```python
from build123d import *

# Parameters (mm, degrees)
SKETCH1_R           = 50
BOSS_EXTRUDE1_DEPTH = 20
CUT_EXTRUDE3_DEPTH  = 74.484692283
SKETCH14_W          = 22.5
SKETCH14_H          = 12.2
CUT_EXTRUDE4_DEPTH  = 74.484692283
SKETCH16_W          = 4.8
SKETCH16_H          = 12.2
CUT_EXTRUDE5_DEPTH  = 11.25
CUT_EXTRUDE7_START  = -11.25
SKETCH17_R          = 0.5
CUT_EXTRUDE7_DEPTH  = 0.4
CUT_EXTRUDE8_DEPTH  = 74.484692283
FILLET1_R           = 2
FILLET2_R           = 0.5
SKETCH4_R           = 14
CUT_EXTRUDE2_DEPTH  = 74.484692283
SKETCH20_W          = 4.8
SKETCH20_H          = 12.2
BOSS_EXTRUDE2_DEPTH = 4
FILLET3_R           = 10


with BuildPart() as part:
    # Sketch1 → Boss-Extrude1 (new body)
    with BuildSketch(Plane(origin=(0, 0, 0), x_dir=(1, 0, 0), z_dir=(0, 1, 0))):
        with Locations(Location((0, 0, 0), (0, 0, 270))):
            Circle(SKETCH1_R)
    extrude(amount=BOSS_EXTRUDE1_DEPTH)

    # Sketch15 → Cut-Extrude3 (cut, through all)
    with BuildSketch(Plane.XZ):
        with BuildLine():
            Line((-21.2, 6.1), (-21.2, 45.283109434))
            ThreePointArc((-21.2, 45.283109434), (-5.873377692, 49.65383605), (10.05, 48.979562064))
            Line((10.05, 48.979562064), (10.9, 6.1))
            Line((10.9, 6.1), (-21.2, 6.1))
        make_face()
    extrude(amount=-CUT_EXTRUDE3_DEPTH, mode=Mode.SUBTRACT)

    # Sketch14 → Cut-Extrude4 (cut, through all)
    with BuildSketch(Plane.XZ):
        with Locations((-5.15, 0)):
            Rectangle(SKETCH14_W, SKETCH14_H)
    extrude(amount=-CUT_EXTRUDE4_DEPTH, mode=Mode.SUBTRACT)

    # Sketch16 → Cut-Extrude5 (cut)
    with BuildSketch(Plane.XZ):
        with Locations((-18.8, 0)):
            Rectangle(SKETCH16_W, SKETCH16_H)
        with Locations((8.5, 0)):
            Rectangle(SKETCH16_W, SKETCH16_H)
    extrude(amount=-CUT_EXTRUDE5_DEPTH, mode=Mode.SUBTRACT)

    # Sketch17 → Cut-Extrude7 (cut)
    with BuildSketch(Plane.XZ.offset(CUT_EXTRUDE7_START)):
        with Locations(Location((8.75, 0, 0), (0, 0, 270))):
            Circle(SKETCH17_R)
        with Locations(Location((-19.05, 0, 0), (0, 0, 270))):
            Circle(SKETCH17_R)
    extrude(amount=-CUT_EXTRUDE7_DEPTH, mode=Mode.SUBTRACT)

    # Sketch18 → Cut-Extrude8 (cut, through all)
    with BuildSketch(Plane(origin=(0, 0, 0), x_dir=(-1, 0, 0), z_dir=(0, -1, 0))):
        with BuildLine():
            Line((-10.9, -6.1), (-49.626505015, -6.1))
            ThreePointArc((-49.626505015, -6.1), (0, -50), (49.626505015, -6.1))
            Line((49.626505015, -6.1), (-10.9, -6.1))
        make_face()
    extrude(amount=-CUT_EXTRUDE8_DEPTH, mode=Mode.SUBTRACT)

    # Fillet1
    fillet1_edges = [part.edges().sort_by_distance(p)[0] for p in [
        (-16.4, 15.625, 6.1),
        (6.1, 15.625, 6.1),
    ]]
    fillet(fillet1_edges, radius=FILLET1_R)

    # Fillet2
    fillet2_edges = [part.edges().sort_by_distance(p)[0] for p in [
        (-19.8, 11.25, 6.1),
        (-16.985786438, 11.25, 5.514213562),
        (6.1, 11.25, -1),
        (6.685786438, 11.25, 5.514213562),
        (-16.4, 11.25, -1),
        (9.5, 11.25, 6.1),
    ]]
    fillet(fillet2_edges, radius=FILLET2_R)

    # Sketch4 → Cut-Extrude2 (cut, through all)
    with BuildSketch(Plane(origin=(0, 20, 0), x_dir=(1, 0, 0), z_dir=(0, 1, 0))):
        with Locations(Location((26.585522376, 13.9, 0), (0, 0, 270))):
            Circle(SKETCH4_R)
    extrude(amount=-CUT_EXTRUDE2_DEPTH, mode=Mode.SUBTRACT)

    # Sketch20 → Boss-Extrude2 (add)
    with BuildSketch(Plane.XZ):
        with Locations((-18.8, 0)):
            Rectangle(SKETCH20_W, SKETCH20_H)
        with Locations((8.5, 0)):
            Rectangle(SKETCH20_W, SKETCH20_H)
    extrude(amount=-BOSS_EXTRUDE2_DEPTH)

    # Fillet3
    fillet3_edges = [part.edges().sort_by_distance(p)[0] for p in [
        (-49.626505015, 10, 6.1),
    ]]
    fillet(fillet3_edges, radius=FILLET3_R)


solid = part.part
```
Model file for the job. Use its own axes, mm. A direction names the side the tool comes from. Give positions to 0.01 mm unless a question says otherwise; leave off trailing zeros. Loops run counter-clockwise (first coordinate to the right, second up) from the corner with the lowest first, then second, coordinate; pieces in that order, holes last. Notation, with made-up numbers: (-8, -25) -> (18, -25) arc R17 ccw to (18, 6) -> close; hole circle Ø11 at (71, 67.25). An arc over 180 degrees is marked (long way). Use CSV: the item, a comma, the result in double quotes. Start each with the question number.
1) Wall check: line 1 (X direction, y = 14, z = -4); line 2 (X direction, y = 12, z = -5); line 3 (X direction, y = 6.75, z = 1). Give the ranges that are in metal, low to high.
2) Tool access for faces 1 (the flat face through (-16.4, 16, -1)), 2 (the cylindrical face through (-16.97, 15.93, 5.5)), 3 (the flat face through (28, 10, 6.1)), 4 (the flat face through (-20, 11.25, 0)): list every direction of +Z, -Z, +X, -X, +Y, -Y with a clear straight run to the whole face (end or side of a thin tool).
3) Mould opens along Y. For faces 5 (the flat face through (-21.2, 7, 0)), 6 (the flat face through (8, 11.25, 0)), 7 (the cylindrical face through (6.7, 15.93, 5.53)), 8 (the flat face through (1, 20, -22)) say: released by +Y, released by -Y, zero draft, split by the parting line, or undercut.
4) Slice it at A-A on z = -13.9. Give the cut face in (x, y).
5) Slice it at C-C on x = 3. Give the cut face in (y, z), plus the area to 3 significant figures.
6) Flat gauge pins, fed straight in: pin 1 Ø6 at (y, z) = (10, -8) entering from +X; pin 2 Ø2 at (y, z) = (1, -2) entering from -X; pin 3 Ø2 at (y, z) = (13, -8.5) entering from +X. Where does each tip first touch, or does it go through?
Computed values:
1,line 1,"x = -49.81 to -16.4, 6.1 to 16.69, 36.48 to 49.84"
1,line 2,"x = -49.75 to -16.4, 6.1 to 15.78, 37.39 to 49.75"
1,line 3,"x = -48.53 to -21.2, 10.9 to 49.99"
2,face 1,"+Z, +Y, -Y"
2,face 2,"+Z, +Y"
2,face 3,"+Z, +X, -X, +Y, -Y"
2,face 4,"+Z"
3,face 5,"undercut"
3,face 6,"undercut"
3,face 7,"zero draft"
3,face 8,"released by +Y"
4,outline,"(-48.03, 0) -> (12.59, 0) -> (12.59, 20) -> (-48.03, 20) -> close; (40.59, 0) -> (48.03, 0) -> (48.03, 20) -> (40.59, 20) -> close"
5,outline,"(0, -49.91) -> (20, -49.91) -> (20, -6.1) -> (0, -6.1) -> close"
5,area,"876 mm^2"
6,pin 1,"stops at x = 49.75"
6,pin 2,"stops at x = -49.77"
6,pin 3,"stops at x = 49.43"
